Read the model definition and answer for the solid it produces. Units are mm, in the model's axes. A direction names the side the tool comes from. Give positions to 0.01 mm unless a question says otherwise; leave off trailing zeros. Order: outer loops, then holes, each group sorted by start corner. A loop starts at its lowest first (then second) coordinate and runs counter-clockwise, first axis right, second up. Notation, with made-up numbers: M -40,-28 L -29,-28 A25 ccw -29,8 Z; hole C 56.5,64 d4. An arc over 180 degrees is marked long. One line per item, written item: value.
from build123d import *

# Parameters (mm, degrees)
SKETCH1_W           = 50
SKETCH1_H           = 5
BOSS_EXTRUDE1_DEPTH = 60
SKETCH2_R           = 3.925
SKETCH2_R_2         = 1.45
CUT_EXTRUDE1_DEPTH  = 6
CHAMFER1_SIZE       = 1.5
FILLET2_R           = 5
SKETCH2_3_W         = 12
SKETCH2_3_H         = 10
SKETCH2_3_R         = 3.8
BOSS_EXTRUDE2_DEPTH = 5
FILLET5_R           = 2.5
FILLET6_R           = 2.5
CHAMFER2_SIZE       = 1.5
CHAMFER3_SIZE       = 1.5


with BuildPart() as part:
    # Sketch1 → Boss-Extrude1 (new body)
    with BuildSketch(Plane(origin=(0, 0, 0), x_dir=(0, 0, -1), z_dir=(1, 0, 0))):
        with Locations((25, 2.5)):
            Rectangle(SKETCH1_W, SKETCH1_H)
    extrude(amount=BOSS_EXTRUDE1_DEPTH)

    # Sketch2 → Cut-Extrude1 (cut, through all)
    with BuildSketch(Plane(origin=(0, 5, 0), x_dir=(1, 0, 0), z_dir=(0, 1, 0))):
        with Locations((49.575, 40.5)):
            Circle(SKETCH2_R)
        with Locations((56, 25)):
            Circle(SKETCH2_R_2)
        with Locations((30, 13.75)):
            Circle(SKETCH2_R_2)
        with Locations((49.575, 9.5)):
            Circle(SKETCH2_R)
        with Locations((10.425, 9.5)):
            Circle(SKETCH2_R)
        with Locations((4, 25)):
            Circle(SKETCH2_R_2)
        with Locations((10.425, 40.5)):
            Circle(SKETCH2_R)
        with Locations((30, 36.25)):
            Circle(SKETCH2_R_2)
    extrude(amount=-CUT_EXTRUDE1_DEPTH, mode=Mode.SUBTRACT)

    # Chamfer1
    chamfer1_edges = [part.edges().sort_by_distance(p)[0] for p in [
        (6.5, 5, -9.5),
        (45.65, 5, -9.5),
        (6.5, 5, -40.5),
        (45.65, 5, -40.5),
    ]]
    chamfer(chamfer1_edges, length=CHAMFER1_SIZE)

    # Fillet2
    fillet2_edges = [part.edges().sort_by_distance(p)[0] for p in [
        (60, 2.5, -50),
        (60, 2.5, 0),
        (0, 2.5, -50),
        (0, 2.5, 0),
    ]]
    fillet(fillet2_edges, radius=FILLET2_R)

    # Sketch2_3 → Boss-Extrude2 (add)
    with BuildSketch(Plane(origin=(0, 5, 0), x_dir=(1, 0, 0), z_dir=(0, 1, 0))):
        with Locations((47.5, 55)):
            Rectangle(SKETCH2_3_W, SKETCH2_3_H)
        with Locations((47.5, 55)):
            Circle(SKETCH2_3_R, mode=Mode.SUBTRACT)
        with Locations((12.5, 55)):
            Rectangle(SKETCH2_3_W, SKETCH2_3_H)
        with Locations((12.5, 55)):
            Circle(SKETCH2_3_R, mode=Mode.SUBTRACT)
        with Locations((47.5, -5)):
            Rectangle(SKETCH2_3_W, SKETCH2_3_H)
        with Locations((47.5, -5)):
            Circle(SKETCH2_3_R, mode=Mode.SUBTRACT)
        with Locations((12.5, -5)):
            Rectangle(SKETCH2_3_W, SKETCH2_3_H)
        with Locations((12.5, -5)):
            Circle(SKETCH2_3_R, mode=Mode.SUBTRACT)
    extrude(amount=-BOSS_EXTRUDE2_DEPTH)

    # Fillet5
    fillet5_edges = [part.edges().sort_by_distance(p)[0] for p in [
        (18.5, 2.5, 10),
        (6.5, 2.5, 10),
        (53.5, 2.5, 10),
        (41.5, 2.5, 10),
        (41.5, 2.5, -60),
        (53.5, 2.5, -60),
        (6.5, 2.5, -60),
        (18.5, 2.5, -60),
    ]]
    fillet(fillet5_edges, radius=FILLET5_R)

    # Fillet6
    fillet6_edges = [part.edges().sort_by_distance(p)[0] for p in [
        (18.5, 2.5, 0),
        (53.5, 2.5, 0),
        (6.5, 2.5, 0),
        (41.5, 2.5, 0),
        (6.5, 2.5, -50),
        (41.5, 2.5, -50),
        (53.5, 2.5, -50),
        (18.5, 2.5, -50),
    ]]
    fillet(fillet6_edges, radius=FILLET6_R)

    # Chamfer2
    chamfer2_edges = [part.edges().sort_by_distance(p)[0] for p in [
        (28.55, 0, -13.75),
        (54.55, 0, -25),
        (28.55, 0, -36.25),
    ]]
    chamfer(chamfer2_edges, length=CHAMFER2_SIZE)

    # Chamfer3
    chamfer3_edges = [part.edges().sort_by_distance(p)[0] for p in [
        (2.55, 0, -25),
    ]]
    chamfer(chamfer3_edges, length=CHAMFER3_SIZE)


solid = part.part
1) Find section B-B, the plane z = -25. Write down the section's boundary in (x, y), plus the area to 4 significant figures.
Reported:
outline: M 0,0 L 1.05,0 L 2.55,1.5 L 2.55,5 L 0,5 Z; M 5.45,1.5 L 6.95,0 L 53.05,0 L 54.55,1.5 L 54.55,5 L 5.45,5 Z; M 57.45,1.5 L 58.95,0 L 60,0 L 60,5 L 57.45,5 Z
area: 266.5 mm^2
2) Find section A-A, the plane x = 30. Write down the section's boundary in (y, z).
Reported:
outline: M 0,-50 L 5,-50 L 5,-37.7 L 1.5,-37.7 L 0,-39.2 Z; M 0,-33.3 L 1.5,-34.8 L 5,-34.8 L 5,-15.2 L 1.5,-15.2 L 0,-16.7 Z; M 0,-10.8 L 1.5,-12.3 L 5,-12.3 L 5,0 L 0,0 Z
3) Consider probe 1 along X at (y, z) = (3.05, 5); probe 2 along Z at (x, y) = (30, 3.45); probe 3 along X at (y, z) = (1.4, -43.5). Determine where each line is inside the solid, lowest interval first.
Reported:
probe 1: x = 6.5 to 8.7, 16.3 to 18.5, 41.5 to 43.7, 51.3 to 53.5
probe 2: z = -50 to -37.7, -34.8 to -15.2, -12.3 to 0
probe 3: x = 0 to 7.89, 12.96 to 47.04, 52.11 to 60
4) Which of the six approach directions +Z, -Z, +X, -X, +Y, -Y give full straight-line access (tool end or side, diameter ignored) to faces 4 (the face through (41, 2, 1)), 5 (the face through (7, 2, 9)), 6 (the face through (6.5, 3, -55))?
Reported:
face 4: +Z, +Y, -Y
face 5: +Z, -X, +Y, -Y
face 6: -Z, -X, +Y, -Y
5) Find section C-C, the plane z = -55. Write down the section's boundary in (x, y).
Reported:
outline: M 6.5,0 L 8.7,0 L 8.7,5 L 6.5,5 Z; M 16.3,0 L 18.5,0 L 18.5,5 L 16.3,5 Z; M 41.5,0 L 43.7,0 L 43.7,5 L 41.5,5 Z; M 51.3,0 L 53.5,0 L 53.5,5 L 51.3,5 Z
6) Determine the mould class of faces 1 (the face through (42, 2, -59)), 2 (the face through (6.5, 3, 5)), 3 (the face through (53, 2, 9)) for opening direction X: +X half, -X half, draft (parallel to the pull), parting line (faces both ways), or undercut.
Reported:
face 1: undercut
face 2: -X half
face 3: +X half
7) Each of these flat-tipped pins is pushed along its axis until it touches: pin 1 Ø6.5 at (x, z) = (49.575, -9.5) entering from +Y; pin 2 Ø2.5 at (x, y) = (28, 3.5) entering from +Z; pin 3 Ø2.5 at (y, z) = (3.5, -54) entering from +X; pin 4 Ø1.5 at (x, y) = (30.5, 2) entering from -Z. Where does it stop, or does it pass through?
Reported:
pin 1: passes through
pin 2: stops at z = 0
pin 3: stops at x = 53.5
pin 4: stops at z = -50
8) Find section D-D, the plane x = 49. Count the separate pieces of the cut face and the enclosed holes in it, plus the area to 3 significant figures.
Reported:
separate pieces: 5
enclosed holes: 0
area: 198 mm^2
